Autodesk Inventor part; units mm, degrees
ref_plane "YZ Plane" through (0, 0, 0) normal (1, 0, 0) x (0, 1, 0)
ref_plane "XZ Plane" through (0, 0, 0) normal (0, 1, 0) x (-1, 0, 0)
ref_plane "XY Plane" through (0, 0, 0) normal (0, 0, 1) x (1, 0, 0)
sketch "Sketch1" plane through (0, 0, 0) normal (0, 0, 1) x (1, 0, 0)
  line L0 (-8.4106, 7.1523) -> (31.5894, 7.1523)
  line L1 (31.5894, 7.1523) -> (31.5894, -32.8477)
  line L2 (31.5894, -32.8477) -> (-8.4106, -32.8477)
  line L3 (-8.4106, -32.8477) -> (-8.4106, 7.1523)
  point P0 (0, 0)
  dimension "d0" = 40
  dimension "d1" = 40
extrude "Plate1" add sketch "Sketch1" along normal blind 0.5
sketch "Sketch2" plane through (0, 0, 0.5) normal (0, 0, 1) x (1, 0, 0)
  line L0 (19.5039, -11.896) -> (5.5039, -11.896) construction
  line L1 (19.5039, -9.896) -> (5.5039, -9.896)
  line L2 (5.5039, -13.896) -> (19.5039, -13.896)
  arc A0 (19.5039, -13.896) -> (19.5039, -9.896) centre (19.5039, -11.896) ccw
  arc A1 (5.5039, -9.896) -> (5.5039, -13.896) centre (5.5039, -11.896) ccw
  point P0 (0, 0)
  point P1 (12.5039, -11.896)
  dimension "LG_C" = 14
  dimension "LT_C" = 4
extrude "Cut1" cut sketch "Sketch2" against normal blind 0.5
equation "\"d5\" = Thickness"
equation "\"d2\" = Thickness"
equation "\"BendRadius\" = Thickness"
equation "\"BendReliefWidth\" = Thickness"
equation "\"BendReliefDepth\" = 0.5 * Thickness"
equation "\"CornerReliefSize\" = 4 * Thickness"
equation "\"MinimumRemnant\" = 2 * Thickness"
equation "\"TransitionRadius\" = BendRadius"
equation "\"JacobiRadiusSize\" = BendRadius"
equation "\"GapSize\" = Thickness"
properties part number "DecupajOvalizat1"
CAD build for the part. Positions are in the model's coordinates, mm. A direction names the side the tool comes from. Coordinates: 2 decimals unless noted, no trailing zeros. Order: outer loops, then holes, each group sorted by start corner. A loop starts at its lowest first (then second) coordinate and runs counter-clockwise, first axis right, second up. Notation, with made-up numbers: M 81.5,15 L 105.5,15 A35 cw 105.5,54 Z; hole C -32.75,24.5 d10. An arc over 180 degrees is marked long. Write each question's results on one line, items separated by ' | '. Start each with the question number.
Q1. Cut at C-C (x = 5). List the corners of the cut face in (y, z).
Q2. Cut at B-B (x = 9.5). List the corners of the cut face in (y, z), then the cut area to 3 significant figures.
Q3. Cut at A-A (z = 0.3). List the corners of the cut face in (x, y), then the cut area to 3 significant figures.
Q4. Pull direction Y, two halves, no side cores. Call faces 1 (the flat face through (11, -8, 0.5)), 2 (the cylindrical face through (21.503, -11.94, 0.254)): +Y half, -Y half, draft (parallel to the pull), parting line (faces both ways), or undercut.
Q5. Which spindle directions (+Z, -Z, +X, -X, +Y, -Y) get a long thin tool onto all of the face, cutting with end or side? Do faces 3 (the cylindrical face through (3.504, -11.852, 0.254)), 4 (the flat face through (11, -8, 0)). Say none if no direction does.
Q6. Drill centre lines: probe 1 along Y at (x, z) = (9, 0.1); probe 2 along Y at (x, z) = (4.5, 0.4); probe 3 along X at (y, z) = (-11, 0.35). Where is each one in solid material? Low to high. Write a range as from..to.
Found:
1) outline: M -32.85,0 L -13.83,0 L -13.83,0.5 L -32.85,0.5 Z; M -9.96,0 L 7.15,0 L 7.15,0.5 L -9.96,0.5 Z
2) outline: M -32.85,0 L -13.9,0 L -13.9,0.5 L -32.85,0.5 Z; M -9.9,0 L 7.15,0 L 7.15,0.5 L -9.9,0.5 Z | area: 18.0 mm²
3) outline: M -8.41,-32.85 L 31.59,-32.85 L 31.59,7.15 L -8.41,7.15 Z; hole M 5.5,-13.9 L 19.5,-13.9 A2 ccw 19.5,-9.9 L 5.5,-9.9 A2 ccw Z | area: 1,530 mm²
4) face 1: draft | face 2: undercut
5) face 3: +Z, -Z | face 4: -Z, +X, -X, +Y, -Y
6) probe 1: -32.85..-13.9, -9.9..7.15 | probe 2: -32.85..-13.63, -10.17..7.15 | probe 3: -8.41..3.72, 21.29..31.59
